Answer from the drawing. Dimensions are ordinates in mm from the lowest x, y and z of the part. A direction names the side the tool comes from. Coordinates: 2 decimals unless noted, no trailing zeros. Order: outer loops, then holes, each group sorted by start corner. A loop starts at its lowest first (then second) coordinate and runs counter-clockwise, first axis right, second up. Notation, with made-up numbers: (46, 13.5) - (79, 13.5) arc R22 cw to (79, 42.5) - close; hole circle Ø5 at (30.25, 69). An arc over 180 degrees is marked (long way). Answer as a JSON object with one key per item and string values. Group by question number.
1) Find the intervals of material crossed by line 1 along Y through (x, z) = (2.25, 25.5); line 2 along X through (y, z) = (1, 2.5); line 3 along Z through (x, y) = (3.75, 4.25), in increasing order.
2) Section A-A (z = 2.5) is taken. Give the vertices of the cut face in (x, y).
3) A tool of negligible diameter and unlimited length cuts with its end or side. For the marked faces 1 and 2, from which of +Z, -Z, +X, -X, +Y, -Y can it reach the whole face along a straight path? Write none if from no direction.
4) Section D-D (y = 6.5) is taken. Give the vertices of the cut face in (x, z), plus the area to 3 significant figures.
5) The mould has two halves that part along Z. Classify the marked faces 3, 4 and 5: released by +Z, released by -Z, zero draft, split by the parting line, or undercut.
6) Section B-B (x = 5) is taken. Give the vertices of the cut face in (y, z), plus the area to 3 significant figures.
7) Each of these flat-tipped pins is pushed along its axis until it touches: P1, Ø1, axis at x = 8.5, z = 11.5, coming from the -Y side; P2, Ø1.6, axis at x = 5, z = 2.5, coming from the +Y side; P3, Ø2, axis at x = 3, y = 5, coming from the +Z side; P4, Ø1.6, axis at x = 6.5, z = 27.5, coming from the +Y side. Where does it stop, or does it pass through?
8) Section C-C (x = 9) is taken. Give the vertices of the cut face in (y, z).
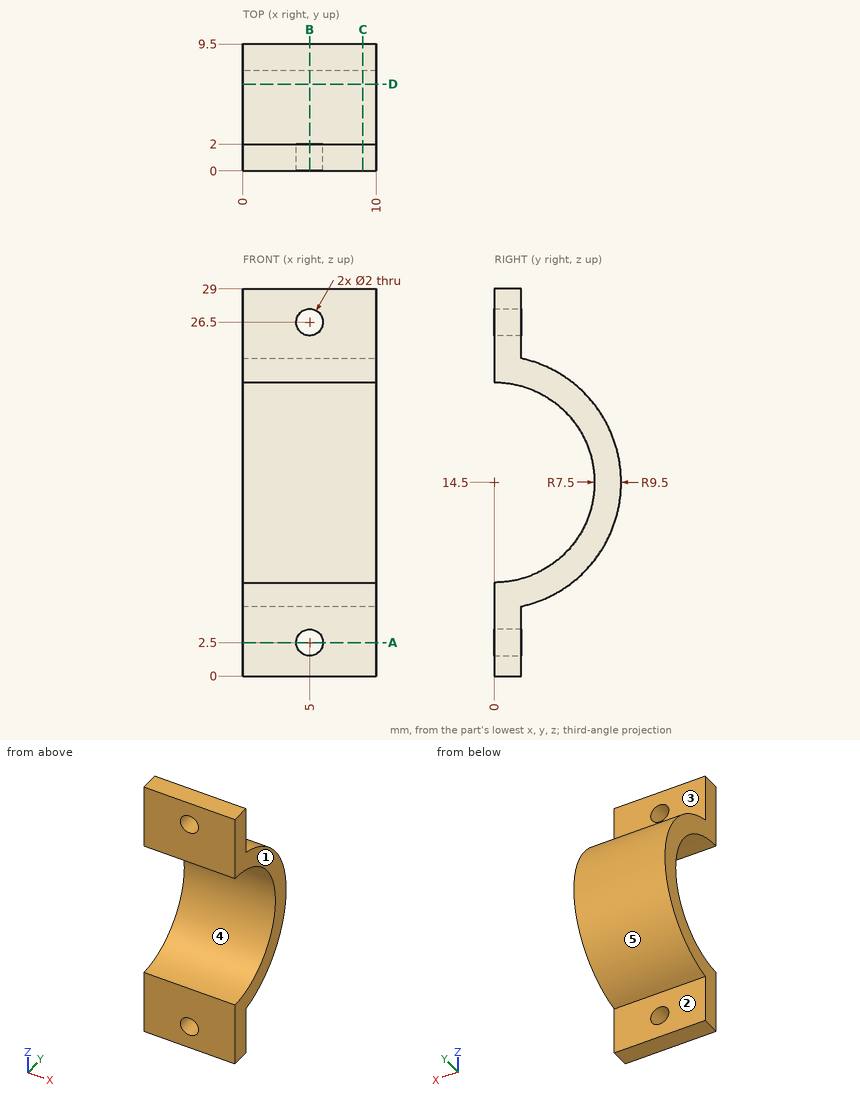
Report:
{
 "1": {"line 1": "y = 0 to 2", "line 2": "x = 0 to 4, 6 to 10", "line 3": "z = 6 to 8.32, 20.68 to 23"},
 "2": {"outline": "(0, 0) - (4, 0) - (4, 2) - (0, 2) - close; (6, 0) - (10, 0) - (10, 2) - (6, 2) - close"},
 "3": {"face 1": "+Z, -Z, +X, +Y, -Y", "face 2": "-Z, +X, -X, +Y"},
 "4": {"outline": "(0, 7.57) - (10, 7.57) - (10, 10.76) - (0, 10.76) - close; (0, 18.24) - (10, 18.24) - (10, 21.43) - (0, 21.43) - close", "area": "63.7 mm²"},
 "5": {"face 3": "zero draft", "face 4": "undercut", "face 5": "split by the parting line"},
 "6": {"outline": "(0, 0) - (2, 0) - (2, 1.5) - (0, 1.5) - close; (0, 3.5) - (2, 3.5) - (2, 5.21) arc R9.5 ccw to (2, 23.79) - (2, 25.5) - (0, 25.5) - (0, 22) arc R7.5 cw to (0, 7) - close; (0, 27.5) - (2, 27.5) - (2, 29) - (0, 29) - close", "area": "65.7 mm²"},
 "7": {"P1": "stops at y = 6.63", "P2": "passes through", "P3": "stops at z = 23.12", "P4": "stops at y = 2"},
 "8": {"outline": "(0, 0) - (2, 0) - (2, 5.21) arc R9.5 ccw to (2, 23.79) - (2, 29) - (0, 29) - (0, 22) arc R7.5 cw to (0, 7) - close"}
}
